```python
from build123d import *

# Parameters (mm, degrees)
F0_R            = 25.4
F1_DEPTH        = 19.05
F2_R            = 27.94
F2_R_2          = 25.4
F3_DEPTH        = 2.54
F5_DEPTH        = 38.1
F5_COPIES_COUNT = 8
F6_R            = 27.94
F7_DEPTH        = 2.54
F8_R            = 3.175
F9_DEPTH        = 43.181


# Not quite as in the source:
# - a pattern or mirror of a feature is missing from the dataset's text; its kind, count and spacing are read off the source's solid


with BuildPart() as f1:
    # F0 (on Top) → F1 (new body, symmetric)
    with BuildSketch(Plane.XY):
        Circle(F0_R)
    extrude(amount=F1_DEPTH, both=True)

    # F2 (on face) → F3 (join)
    with BuildSketch(Plane.XY.offset(19.05)):
        Circle(F2_R)
        Circle(F2_R_2, mode=Mode.SUBTRACT)
        Circle(F2_R_2)
    extrude(amount=F3_DEPTH)

    # F4 (on face) → F5 (cut, through all)
    with BuildSketch(Plane(origin=(0, 0, -19.05), x_dir=(1, 0, 0), z_dir=(0, 0, -1))):
        with BuildLine():
            ThreePointArc((4.1803474687, 25.0536363636), (0, 25.4), (-4.1803474687, 25.0536363636))
            ThreePointArc((-4.1803474687, 25.0536363636), (0, 22.86), (4.1803474687, 25.0536363636))
        make_face()
    f5 = extrude(amount=-F5_DEPTH, mode=Mode.SUBTRACT)

    # F5_copies: F5 ×8 about axis
    f5_copies_axis = Axis((0, 0, 0), (0, 0, 1))
    for i in range(1, F5_COPIES_COUNT):
        add(f5.rotate(f5_copies_axis, i * 360 / F5_COPIES_COUNT), mode=Mode.SUBTRACT)

    # F6 (on face) → F7 (join)
    with BuildSketch(Plane(origin=(0, 0, -19.05), x_dir=(1, 0, 0), z_dir=(0, 0, -1))):
        Circle(F6_R)
    extrude(amount=F7_DEPTH)

    # F8 (on face) → F9 (cut, through all)
    with BuildSketch(Plane(origin=(0, 0, -21.59), x_dir=(1, 0, 0), z_dir=(0, 0, -1))):
        Circle(F8_R)
    extrude(amount=-F9_DEPTH, mode=Mode.SUBTRACT)


solid = f1.part
```
Check sheet for the modelled part. Datum: model origin and axes. Units: mm. A direction names the side the tool comes from. Give positions to 0.01 mm unless a question says otherwise; leave off trailing zeros. Write each loop counter-clockwise with the first axis right and the second up, starting at its lowest first coordinate (ties: lowest second). Pieces come first, ordered by that corner, then holes.
Item 1: Cross-section at A-A (x = 0). Enter the section's corners in (y, z) (3 decimals), and give its area (3 significant figures).
Item 2: Draft check along Y on faces 6 (the face through (22.86, -0.07, -0.27)), 7 (the face through (23.435, -9.795, 0.267)), 8 (the face through (-3.64, 27.7, 20.3)), 9 (the face through (0.07, 22.86, -0.27)). Enter one of: released by +Y, released by -Y, zero draft, split by the parting line, or undercut.
Item 3: Access from +Z, -Z, +X, -X, +Y, -Y to the whole of each face (thin tool, end or side, straight path). Record for faces 1 (the face through (-9.645, 23.497, 0.267)), 2 (the face through (23.497, 9.645, 0.267)), 3 (the face through (16.12, -16.21, -0.27)), 4 (the face through (-9.795, -23.435, 0.267)), 5 (the face through (-3.64, -27.7, -20.3)).
Item 4: Cross-section at C-C (z = 10.5). Enter the section's corners in (x, y) (3 decimals).
Item 5: Cross-section at D-D (x = 15.5). Enter the section's corners in (y, z).
Item 6: Gauge pin test, flat ends, axial feed: pin 1 (12 mm diameter, centred on y = -2.5, z = -12.5, fed in from +X); pin 2 (8 mm diameter, centred on y = -21.5, z = 13, fed in from -X); pin 3 (5 mm diameter, centred on x = 11.5, z = 10.5, fed in from -Y); pin 4 (5.5 mm diameter, centred on x = 0, y = 0, fed in from +Z). Record the tip position at first contact, or that the pin passes through.
Item 7: Scan lines: L1, parallel to X at y = 0, z = 8 (3 decimals); L2, parallel to Z at x = -19, y = 19. Record each from-to range of solid material in increasing order.
Report:
1. outline: (-27.94, -21.59) - (-3.175, -21.59) - (-3.175, 21.59) - (-27.94, 21.59) - (-27.94, 19.05) - (-22.86, 19.05) - (-22.86, -19.05) - (-27.94, -19.05) - close; (3.175, -21.59) - (27.94, -21.59) - (27.94, -19.05) - (22.86, -19.05) - (22.86, 19.05) - (27.94, 19.05) - (27.94, 21.59) - (3.175, 21.59) - close
1. area: 1,750 mm2
2. face 6: undercut
2. face 7: released by -Y
2. face 8: split by the parting line
2. face 9: released by +Y
3. face 1: -X, +Y
3. face 2: +X, +Y
3. face 3: none
3. face 4: -X, -Y
3. face 5: +Z, -Z
4. outline: (-25.054, -4.18) arc R25.4 ccw to (-20.672, -14.76) arc R5.08 cw to (-14.76, -20.672) arc R25.4 ccw to (-4.18, -25.054) arc R5.08 cw to (4.18, -25.054) arc R25.4 ccw to (14.76, -20.672) arc R5.08 cw to (20.672, -14.76) arc R25.4 ccw to (25.054, -4.18) arc R5.08 cw to (25.054, 4.18) arc R25.4 ccw to (20.672, 14.76) arc R5.08 cw to (14.76, 20.672) arc R25.4 ccw to (4.18, 25.054) arc R5.08 cw to (-4.18, 25.054) arc R25.4 ccw to (-14.76, 20.672) arc R5.08 cw to (-20.672, 14.76) arc R25.4 ccw to (-25.054, 4.18) arc R5.08 cw to start; hole circle Ø6.35 at (0, 0)
5. outline: (-23.25, -21.59) - (23.25, -21.59) - (23.25, -19.05) - (16.98, -19.05) - (16.98, 19.05) - (23.25, 19.05) - (23.25, 21.59) - (-23.25, 21.59) - (-23.25, 19.05) - (-16.98, 19.05) - (-16.98, -19.05) - (-23.25, -19.05) - close
6. pin 1: stops at x = 25.05
6. pin 2: stops at x = -15.21
6. pin 3: stops at y = -23.75
6. pin 4: passes through
7. L1: x = -22.86 to -3.175, 3.175 to 22.86
7. L2: z = -21.59 to -19.05, 19.05 to 21.59
